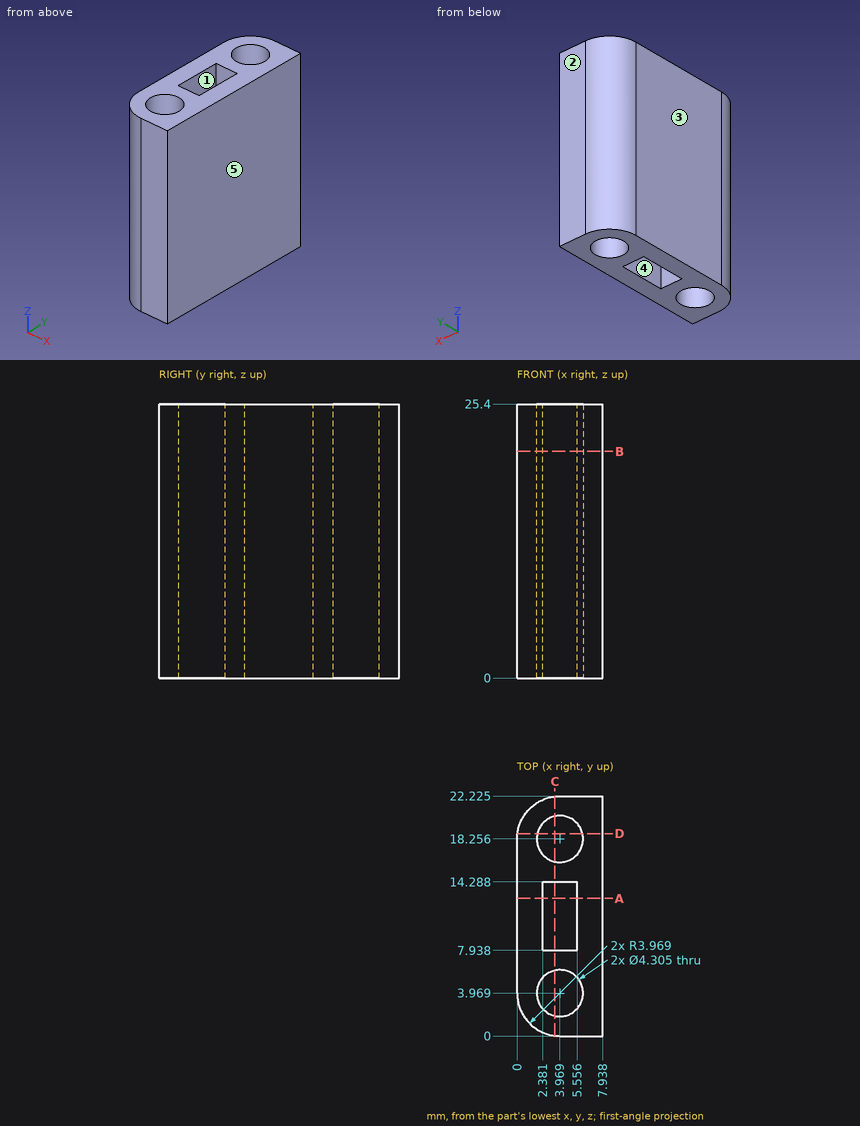
Geometry: see drawing. Coordinates: mm, zero at the bounding-box minimum. A direction names the side the tool comes from. Coordinates: 2 decimals unless noted, no trailing zeros. Order: outer loops, then holes, each group sorted by start corner. A loop starts at its lowest first (then second) coordinate and runs counter-clockwise, first axis right, second up. Notation, with made-up numbers: M 55,5.25 L 70,5.25 A17 ccw 70,18.25 Z; hole C 88,56.25 d3. An arc over 180 degrees is marked long. Answer in a Markdown table with one row per item. Add a question column.
Q1. Reachability of the marked faces 4 and 5 from +Z, -Z, +X, -X, +Y, -Y: full face, straight path, thin tool, end or side. Return the list, or none.
Q2. Contact query for flat-ended pins moving along their axis: P1, Ø2, axis at y = 3.5, z = 10.5, coming from the -X side; P2, Ø2.5, axis at x = 3.97, y = 18.26, coming from the -Z side. Output: stop coordinate, or through.
Q3. Section query C-C on x = 3.5. Return the cut outline in (y, z) (1 decimal).
Q4. Section query D-D on y = 18.75. Return the cut outline in (x, z) (1 decimal).
Q5. Line query: L1, parallel to Y at x = 4, z = 6 (1 decimal); L2, parallel to X at y = 14.25, z = 6.75; L3, parallel to Y at x = 2.75, z = 21 (1 decimal). Output: solid intervals per line, ascending.
Q6. Section query A-A on y = 12.75. Return the cut outline in (x, z), and give its area (3 significant figures).
Q7. Section query B-B on z = 21. Return the cut outline in (x, y) (1 decimal).
Q8. Mould query, pull axis X, two halves, no side actions, for the marked faces 1, 2 and 3. Classes: released by +X, released by -X, zero draft, split by the parting line, or undercut.
Completed:
| question | item | result |
|---|---|---|
| 1 | face 4 | +Z, -Z |
| 1 | face 5 | +Z, -Z, +X, +Y, -Y |
| 2 | P1 | stops at x = 0 |
| 2 | P2 | passes through |
| 3 | outline | M 0,0 L 1.9,0 L 1.9,25.4 L 0,25.4 Z; M 6.1,0 L 7.9,0 L 7.9,25.4 L 6.1,25.4 Z; M 14.3,0 L 16.2,0 L 16.2,25.4 L 14.3,25.4 Z; M 20.4,0 L 22.2,0 L 22.2,25.4 L 20.4,25.4 Z |
| 4 | outline | M 0,0 L 1.9,0 L 1.9,25.4 L 0,25.4 Z; M 6.1,0 L 7.9,0 L 7.9,25.4 L 6.1,25.4 Z |
| 5 | L1 | y = 0 to 1.8, 6.1 to 7.9, 14.3 to 16.1, 20.4 to 22.2 |
| 5 | L2 | x = 0 to 2.38, 5.56 to 7.94 |
| 5 | L3 | y = 0.2 to 2.2, 5.7 to 7.9, 14.3 to 16.5, 20 to 22 |
| 6 | outline | M 0,0 L 2.38,0 L 2.38,25.4 L 0,25.4 Z; M 5.56,0 L 7.94,0 L 7.94,25.4 L 5.56,25.4 Z |
| 6 | area | 121 mm2 |
| 7 | outline | M 0,4 A4 ccw 4,0 L 7.9,0 L 7.9,22.2 L 4,22.2 A4 ccw 0,18.3 Z; hole C 4,4 d4.3; hole C 4,18.3 d4.3; hole M 2.4,7.9 L 5.6,7.9 L 5.6,14.3 L 2.4,14.3 Z |
| 8 | face 1 | undercut |
| 8 | face 2 | zero draft |
| 8 | face 3 | released by -X |
